Here's the drawing with two shaded views (mm, measured from the low corner). I have some questions. Round coordinates to 2 decimals unless told otherwise and drop trailing zeros. Order: outer loops, then holes, each group sorted by start corner. A loop starts at its lowest first (then second) coordinate and runs counter-clockwise, first axis right, second up. Notation, with made-up numbers: (0, -25) -> (57, -25) arc R11 ccw to (57, -6) -> close; hole circle Ø8 at (1.5, 8.25). An arc over 180 degrees is marked (long way). Answer in a Markdown table with one row per item.
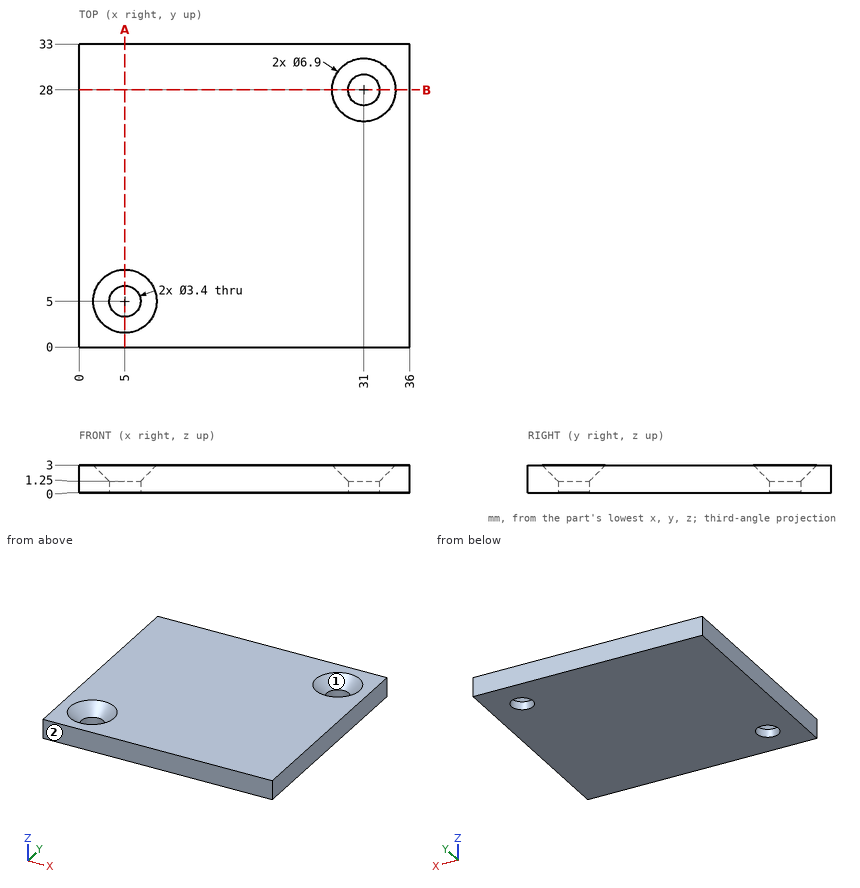
1. Suppose I cut it at B-B on y = 28. Write out the boundary of the cut face in (x, z), then the cut area to 3 significant figures.
Numbers:
| item | result |
|---|---|
| outline | (0, 0) -> (29.3, 0) -> (29.3, 1.25) -> (27.55, 3) -> (0, 3) -> close; (32.7, 0) -> (36, 0) -> (36, 3) -> (34.45, 3) -> (32.7, 1.25) -> close |
| area | 94.7 mm2 |
2. We'd pull the mould along X, two halves only. Please class the marked faces 1 and 2: released by +X, released by -X, zero draft, split by the parting line, or undercut.
Numbers:
| item | result |
|---|---|
| face 1 | undercut |
| face 2 | zero draft |
3. Please list where these lines run through material, in increasing order: line 1 along Y through (x, z) = (31, 0.7); line 2 along Y through (x, z) = (5, 0.9); line 3 along X through (y, z) = (5, 0.95).
Numbers:
| item | result |
|---|---|
| line 1 | y = 0 to 26.3, 29.7 to 33 |
| line 2 | y = 0 to 3.3, 6.7 to 33 |
| line 3 | x = 0 to 3.3, 6.7 to 36 |
4. Suppose I cut it at A-A on x = 5. Write out the boundary of the cut face in (y, z).
Numbers:
| item | result |
|---|---|
| outline | (0, 0) -> (3.3, 0) -> (3.3, 1.25) -> (1.55, 3) -> (0, 3) -> close; (6.7, 0) -> (33, 0) -> (33, 3) -> (8.45, 3) -> (6.7, 1.25) -> close |
5. For pin 1 Ø5.5 at (x, y) = (5, 5) entering from +Z, with a flat end and sliding along its axis, tell me the tip position at first contact or that it passes through.
Numbers:
| item | result |
|---|---|
| pin 1 | stops at z = 2.3 |
